Answer from the drawing. Dimensions are ordinates in mm from the lowest x, y and z of the part. Round coordinates to 2 decimals unless told otherwise and drop trailing zeros. Loops run counter-clockwise (first coordinate to the right, second up) from the corner with the lowest first, then second, coordinate; pieces in that order, holes last. Notation, with made-up numbers: (78.5, 6.5) - (116.5, 6.5) arc R11 ccw to (116.5, 12.5) - close; hole circle Ø2 at (-17.75, 74.25). An arc over 180 degrees is marked (long way). Answer as CSV lines item,"result".
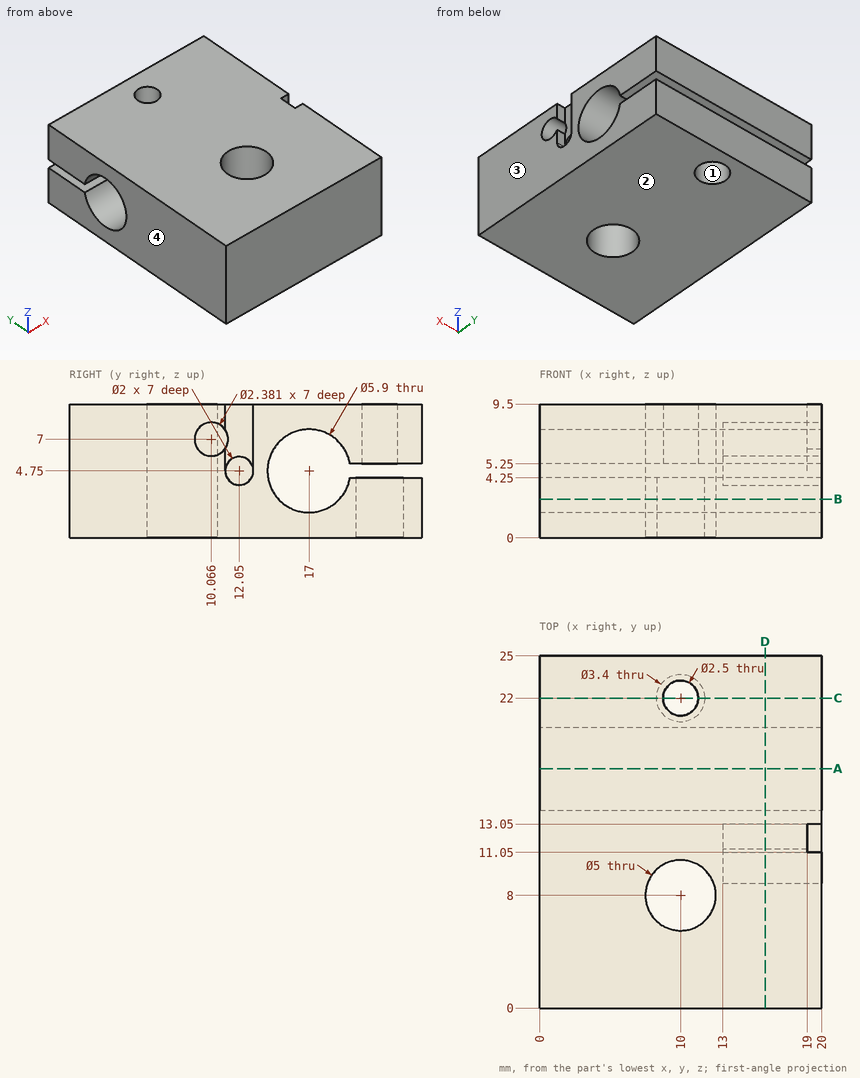
1) The mould has two halves that part along X. Classify the marked faces 1, 2, 3 and 4: pulls with the +X half, pulls with the -X half, needs draft (parallel to the pull), parting line crosses it, or undercut.
Entries:
face 1,"undercut"
face 2,"needs draft"
face 3,"pulls with the +X half"
face 4,"pulls with the -X half"
2) A cutting plane is placed at B-B, the plane z = 2.75. Determine the outline of the cut face in (x, y).
Entries:
outline,"(0, 0) - (20, 0) - (20, 14.83) - (0, 14.83) - close; (0, 19.17) - (20, 19.17) - (20, 25) - (0, 25) - close; hole circle Ø5 at (10, 8); hole circle Ø3.4 at (10, 22)"
3) This flat-tipped pin is pushed along its axis until it touches: P1, Ø0.6, axis at y = 12.5, z = 7, coming from the +X side. Where does it stop, or does it pass through?
Entries:
P1,"stops at x = 19"
4) Find the intervals of material crossed by line 1 (Z direction, x = 19, y = 10); line 2 (X direction, y = 22, z = 7.55); line 3 (Y direction, x = 11.75, z = 3.5) (1 decimal), in increasing order.
Entries:
line 1,"z = 0 to 5.81, 8.19 to 9.5"
line 2,"x = 0 to 8.75, 11.25 to 20"
line 3,"y = 0 to 6.2, 9.8 to 14.3, 19.7 to 25"
5) A cutting plane is placed at A-A, the plane y = 17. Determine the outline of the cut face in (x, z).
Entries:
outline,"(0, 0) - (20, 0) - (20, 1.8) - (0, 1.8) - close; (0, 7.7) - (20, 7.7) - (20, 9.5) - (0, 9.5) - close"
6) A cutting plane is placed at D-D, the plane x = 16. Determine the outline of the cut face in (y, z).
Entries:
outline,"(0, 0) - (25, 0) - (25, 4.25) - (19.91, 4.25) arc R2.95 cw (long way) to (19.91, 5.25) - (25, 5.25) - (25, 9.5) - (0, 9.5) - close; hole circle Ø2.38 at (10.07, 7); hole circle Ø2 at (12.05, 4.75)"
7) A cutting plane is placed at C-C, the plane y = 22. Determine the outline of the cut face in (x, z), plus the area to 3 significant figures.
Entries:
outline,"(0, 0) - (8.3, 0) - (8.3, 4.25) - (0, 4.25) - close; (0, 5.25) - (8.75, 5.25) - (8.75, 9.5) - (0, 9.5) - close; (11.25, 5.25) - (20, 5.25) - (20, 9.5) - (11.25, 9.5) - close; (11.7, 0) - (20, 0) - (20, 4.25) - (11.7, 4.25) - close"
area,"145 mm^2"
